Autodesk Inventor part; units mm, degrees
ref_plane "Work Plane1" through (0, 12, 0) normal (0, 1, 0) x (1, 0, 0)
ref_plane "YZ Plane" through (0, 0, 0) normal (1, 0, 0) x (0, 1, 0)
ref_plane "XZ Plane" through (0, 0, 0) normal (0, 1, 0) x (-1, 0, 0)
sketch "Sketch1" plane through (0, 0, 0) normal (0, 1, 0) x (-1, 0, 0)
  line L0 (27, 44) -> (-27, 44)
  line L1 (-27, 44) -> (-27, -44)
  line L2 (-27, -44) -> (27, -44)
  line L3 (27, -44) -> (27, 44)
  line L4 (27, 44) -> (-27, -44) construction
  line L5 (-27, 44) -> (27, -44) construction
  circle A0 centre (22.3059, 39.9545) radius 2
  circle A1 centre (-22.0879, 39.9545) radius 2
  circle A2 centre (-21.9299, -40.0455) radius 2
  circle A3 centre (22.3059, -40.0455) radius 2
  point P0 (0, 0)
  dimension "d0" = 54
  dimension "d6" = 4
  dimension "d7" = 4
  dimension "d8" = 4
  dimension "d9" = 4
  dimension "d17" = 88
  dimension "d19" = 80
extrude "Extrusion1" add sketch "Sketch1" along normal blind 12
ref_plane "Work Plane1" through (0, 12, 0) normal (0, 1, 0) x (1, 0, 0)
sketch "Sketch2" plane through (0, 12, 0) normal (0, 1, 0) x (1, 0, 0)
  circle A0 centre (11, 20) radius 10
  point P0 (0, 0)
  dimension "d14" = 20
extrude "Extrusion2" add sketch "Sketch2" along normal blind 48
fillet "Fillet1" radius 2 4 edges at (27, 6, 44) (27, 6, -44) (-27, 6, 44) (-27, 6, -44)
properties part number "sensor 2"
Geometry check sheet. Reference: the model listing, model coordinates, mm. A direction names the side the tool comes from. Round coordinates to 2 decimals unless told otherwise and drop trailing zeros. Order: outer loops, then holes, each group sorted by start corner. A loop starts at its lowest first (then second) coordinate and runs counter-clockwise, first axis right, second up. Notation, with made-up numbers: (-12, -36) - (21, -36) arc R18 ccw to (21, -31) - close; hole circle Ø7 at (10, 20). An arc over 180 degrees is marked (long way). Use a Markdown table: item, result. Add a question column.
(1) Sectioned sample at B-B, the plane x = 11. Enter the section's corners in (y, z), and give its area (3 significant figures).
(2) Material ranges on line 1 along Z through (x, y) = (21, 4.5); line 2 along Y through (x, z) = (14.5, -10); line 3 along Z through (x, y) = (18, 50.5), recorded low to high. Write a range as [from, to].
(3) Sectioned sample at C-C, the plane y = 13. Enter the section's corners in (x, z), and give its area (3 significant figures).
(4) Sectioned sample at A-A, the plane z = -20. Enter the section's corners in (x, y), and give its area (3 significant figures).
(5) Tool access check on faces 4 (the cylindrical face through (20.85, 5.92, -41.73)), 5 (the cylindrical face through (3.63, 35.66, -13.24)). Record the directions out of +Z, -Z, +X, -X, +Y, -Y that give a thin tool (end or side, any length) a straight path to the whole face; none if there is none.
(6) Sectioned sample at D-D, the plane z = 0.5. Enter the section's corners in (x, y), and give its area (3 significant figures).
(7) Depth check by flat-ended pin: pin 1 (5 mm diameter, centred on x = -22.31, z = 39.95, fed in from +Y); pin 2 (6.5 mm diameter, centred on x = 22.09, z = 39.95, fed in from -Y); pin 3 (5 mm diameter, centred on x = 5, y = 44, fed in from -Z); pin 4 (10 mm diameter, centred on y = 32, z = -19.5, fed in from +X). Enter the tip coordinate at first touch or a pass-through.
(8) Release check for a two-part mould opening along X. For faces 1 (the flat face through (-27, 6, -1)), 2 (the flat face through (0, 12, 1)), 3 (the cylindrical face through (-22.05, 5.92, 37.97)) record: pulls with the +X half, pulls with the -X half, needs draft (parallel to the pull), parting line crosses it, or undercut.
Answers below:
| question | item | result |
|---|---|---|
| 1 | outline | (0, -44) - (12, -44) - (12, -30) - (60, -30) - (60, -10) - (12, -10) - (12, 44) - (0, 44) - close |
| 1 | area | 2,020 mm² |
| 2 | line 1 | [-44, -41.82], [-38.27, 38.28], [41.63, 44] |
| 2 | line 2 | [0, 12] |
| 2 | line 3 | [-27.14, -12.86] |
| 3 | outline | circle Ø20 at (11, -20) |
| 3 | area | 314 mm² |
| 4 | outline | (-27, 0) - (27, 0) - (27, 12) - (21, 12) - (21, 60) - (1, 60) - (1, 12) - (-27, 12) - close |
| 4 | area | 1,610 mm² |
| 5 | face 4 | +Y, -Y |
| 5 | face 5 | +Y |
| 6 | outline | (-27, 0) - (27, 0) - (27, 12) - (-27, 12) - close |
| 6 | area | 648 mm² |
| 7 | pin 1 | y = 12 |
| 7 | pin 2 | y = 0 |
| 7 | pin 3 | z = -29.37 |
| 7 | pin 4 | x = 21 |
| 8 | face 1 | pulls with the -X half |
| 8 | face 2 | needs draft |
| 8 | face 3 | undercut |
